```python
from build123d import *

# Parameters (mm, degrees)
BOSS_EXTRUDE1_DEPTH = 4
SKETCH2_R           = 2.25
CUT_EXTRUDE1_DEPTH  = 4
SKETCH3_R           = 3
CUT_EXTRUDE2_DEPTH  = 2
CHAMFER1_SIZE       = 1


with BuildPart() as part:
    # Sketch1 → Boss-Extrude1 (new body)
    with BuildSketch(Plane.XY):
        with BuildLine():
            Line((-3.399881961, 2.8), (-3.399881961, -2.8))
            add(Edge.make_bspline(
                [(-3.399881961, -2.8), (-3.399881961, -2.953071187), (-3.271882834, -3.271984466), (-2.952966029, -3.4), (-2.799893385, -3.4)],
                knots=[-1.570796327, -1.570796327, -1.570796327, -1.570796327, -0.785398163, 0, 0, 0, 0], degree=3))
            Line((-2.799893385, -3.4), (2.799893385, -3.4))
            add(Edge.make_bspline(
                [(2.799893385, -3.4), (2.952966029, -3.4), (3.271882834, -3.271984466), (3.399881961, -2.953071187), (3.399881961, -2.8)],
                knots=[0, 0, 0, 0, 0.785398163, 1.570796327, 1.570796327, 1.570796327, 1.570796327], degree=3))
            Line((3.399881961, -2.8), (3.399881961, 2.8))
            add(Edge.make_bspline(
                [(3.399881961, 2.8), (3.399881961, 2.953071187), (3.271882834, 3.271984466), (2.952966029, 3.4), (2.799893385, 3.4)],
                knots=[1.570796327, 1.570796327, 1.570796327, 1.570796327, 2.35619449, 3.141592654, 3.141592654, 3.141592654, 3.141592654], degree=3))
            Line((2.799893385, 3.4), (-2.799893385, 3.4))
            add(Edge.make_bspline(
                [(-2.799893385, 3.4), (-2.952966029, 3.4), (-3.271882834, 3.271984466), (-3.399881961, 2.953071187), (-3.399881961, 2.8)],
                knots=[-3.141592654, -3.141592654, -3.141592654, -3.141592654, -2.35619449, -1.570796327, -1.570796327, -1.570796327, -1.570796327], degree=3))
        make_face()
    extrude(amount=BOSS_EXTRUDE1_DEPTH)

    # Sketch2 → Cut-Extrude1 (cut)
    with BuildSketch(Plane.XY.offset(4)):
        Circle(SKETCH2_R)
    extrude(amount=-CUT_EXTRUDE1_DEPTH, mode=Mode.SUBTRACT)

    # Sketch3 → Cut-Extrude2 (cut)
    with BuildSketch(Plane(origin=(0, 0, 0), x_dir=(-1, 0, 0), z_dir=(0, 0, -1))):
        Circle(SKETCH3_R)
    extrude(amount=-CUT_EXTRUDE2_DEPTH, mode=Mode.SUBTRACT)

    # Chamfer1
    # the kernel refuses this chamfer: 1 mm, written as the material it takes off along each edge
    with BuildSketch(Plane(origin=(0, 0, 2), x_dir=(1, 0, 0), z_dir=(0, -1, 0))) as chamfer1_piece_1_section:
        Polygon((2.25, CHAMFER1_SIZE), (2.25 + CHAMFER1_SIZE, 0), (2.25, 0), align=None)
    chamfer1_piece_1 = revolve(axis=Axis((0, 0, 2), (0, 0, 1)), mode=Mode.PRIVATE)
    chamfer1_piece_1 = chamfer1_piece_1 & Plane(origin=(0, 0, 2.624934748), x_dir=(-1, 0, 0), z_dir=(0, 0, -1)) * Cylinder(3, 13, mode=Mode.PRIVATE)
    add(chamfer1_piece_1, mode=Mode.SUBTRACT)


solid = part.part
```
Geometry check sheet. Reference: the model listing, model coordinates, mm. Give positions to 0.01 mm unless a question says otherwise; leave off trailing zeros. Write each loop counter-clockwise with the first axis right and the second up, starting at its lowest first coordinate (ties: lowest second). Pieces come first, ordered by that corner, then holes.
1) Release check for a two-part mould opening along X. For faces 1 (the flat face through (-2.3, 0.8, 4)), 2 (the flat face through (3.4, 0, 2)), 3 (the cylindrical face through (3, 0, 1)), 4 (the flat face through (-3.4, 0, 2)) record: pulls with the +X half, pulls with the -X half, needs draft (parallel to the pull), parting line crosses it, or undercut.
2) Material ranges on L1, parallel to Y at x = 0, z = 3.6; L2, parallel to X at y = 0, z = 0.75, recorded low to high.
3) Section check A-A, the plane y = 0. Record the boundary of the cut face in (x, z), and give its area (3 significant figures).
Computed:
1. face 1: needs draft
1. face 2: pulls with the +X half
1. face 3: undercut
1. face 4: pulls with the -X half
2. L1: y = -3.4 to -2.25, 2.25 to 3.4
2. L2: x = -3.4 to -3, 3 to 3.4
3. outline: (-3.4, 0) - (-3, 0) - (-3, 2.25) - (-2.25, 3) - (-2.25, 4) - (-3.4, 4) - close; (2.25, 3) - (3, 2.25) - (3, 0) - (3.4, 0) - (3.4, 4) - (2.25, 4) - close
3. area: 5.26 mm2
